from build123d import *

# Parameters (mm, degrees)
BOX016_W     = 3
BOX016_H     = 1
BOX016_DEPTH = 3
BOX015_W     = 1
BOX015_H     = 9
BOX015_DEPTH = 9
BOX014_W     = 3
BOX014_H     = 1
BOX014_DEPTH = 9


with BuildPart() as box016:
    # Box016 → Box016 (new body)
    with BuildSketch(Plane(origin=(27, 15, 7), x_dir=(1, 0, 0), z_dir=(0, 0, 1))):
        with Locations((1.5, 0.5)):
            Rectangle(BOX016_W, BOX016_H)
    extrude(amount=BOX016_DEPTH)


with BuildPart() as box015:
    # Box015 → Box015 (new body)
    with BuildSketch(Plane(origin=(26, 15, 1), x_dir=(1, 0, 0), z_dir=(0, 0, 1))):
        with Locations((0.5, 4.5)):
            Rectangle(BOX015_W, BOX015_H)
    extrude(amount=BOX015_DEPTH)


with BuildPart() as fusion:
    # Box014 → Box014 (new body)
    with BuildSketch(Plane(origin=(30, 15, 1), x_dir=(1, 0, 0), z_dir=(0, 0, 1))):
        with Locations((1.5, 0.5)):
            Rectangle(BOX014_W, BOX014_H)
    extrude(amount=BOX014_DEPTH)

    # Fusion: union Box016, Box015
    add(box016.part)
    add(box015.part)


with BuildPart() as fusion_1:
    # Fusion placement: moved
    add(fusion.part.moved(Location((11, 0, 0))))


solid = fusion_1.part
The model under review builds one solid part; all positions refer to its coordinate system, in mm. A direction names the side the tool comes from. Give positions to 0.01 mm unless a question says otherwise; leave off trailing zeros. Order: outer loops, then holes, each group sorted by start corner. A loop starts at its lowest first (then second) coordinate and runs counter-clockwise, first axis right, second up. Notation, with made-up numbers: M -33,-33 L 13,-33 A25 cw 13,-7 Z; hole C -8.75,-3 d11. An arc over 180 degrees is marked long. Answer in a Markdown table with one row per item. Add a question column.
1. Add section A-A on z = 5.5. State the section outline as (x, y) points, plus the area to 3 significant figures.
2. For pin 1 Ø1 at (x, z) = (41, 5) entering from +Y; pin 2 Ø4.5 at (y, z) = (21, 6) entering from +X; pin 3 Ø3 at (x, y) = (38.5, 19.5) entering from -Z, all flat-tipped, find the tip position at first contact; note any pin that passes through.
3. Add section D-D on x = 43.75. State the section outline as (y, z) points.
4. To check wall thickness, follow line 1 along X through (y, z) = (19.75, 9.25); line 2 along Y through (x, z) = (39, 7.75). State the ranges of each line that lie inside material, in increasing order.
5. Machinability: for faces 1 (the flat face through (41, 15.5, 4)), 2 (the flat face through (42, 16, 6)), 3 (the flat face through (44, 15.5, 5.4)), which of the approach directions +Z, -Z, +X, -X, +Y, -Y give a long, thin tool a straight path to every point of the face, cutting with its end or side? Answer none if there is none.
6. Add section B-B on z = 7.5. State the section outline as (x, y) points, plus the area to 3 significant figures.
7. Add section C-C on y = 23. State the section outline as (x, z) points, plus the area to 3 significant figures.
The answers:
| question | item | result |
|---|---|---|
| 1 | outline | M 37,15 L 38,15 L 38,24 L 37,24 Z; M 41,15 L 44,15 L 44,16 L 41,16 Z |
| 1 | area | 12.0 mm2 |
| 2 | pin 1 | y = 16 |
| 2 | pin 2 | x = 38 |
| 2 | pin 3 | z = 1 |
| 3 | outline | M 15,1 L 16,1 L 16,10 L 15,10 Z |
| 4 | line 1 | 37 to 38 |
| 4 | line 2 | 15 to 16 |
| 5 | face 1 | -Z, +Y, -Y |
| 5 | face 2 | +Z, -Z, +X, +Y |
| 5 | face 3 | +Z, -Z, +X, +Y, -Y |
| 6 | outline | M 37,15 L 44,15 L 44,16 L 38,16 L 38,24 L 37,24 Z |
| 6 | area | 15.0 mm2 |
| 7 | outline | M 37,1 L 38,1 L 38,10 L 37,10 Z |
| 7 | area | 9.00 mm2 |
